from build123d import *

# Parameters (mm, degrees)
F0_W     = 35.4
F0_H     = 23.6
F1_DEPTH = 20
F3_DEPTH = 10


with BuildPart() as f1:
    # F0 (on Front) → F1 (new body)
    with BuildSketch(Plane.XZ):
        with Locations((-17.7, 28)):
            Rectangle(F0_W, F0_H)
        with BuildLine():
            ThreePointArc((0, -39.8), (39.8, 0), (0, 39.8))
            Line((0, 39.8), (0, 16.2))
            ThreePointArc((0, 16.2), (16.2, 0), (0, -16.2))
            Line((0, -16.2), (0, -39.8))
        make_face()
        with Locations((-17.7, -28)):
            Rectangle(F0_W, F0_H)
    extrude(amount=F1_DEPTH)

    # F2 (on face) → F3 (cut)
    with BuildSketch(Plane.XZ.offset(20)):
        with BuildLine():
            ThreePointArc((12.98208, 26.520214), (7.568156, 28.540833), (1.864359, 29.468293))
            ThreePointArc((1.864359, 29.468293), (-0.019794, 27.808362), (1.640137, 25.924209))
            ThreePointArc((1.640137, 25.924209), (6.657951, 25.108293), (11.420755, 23.330688))
            ThreePointArc((11.420755, 23.330688), (13.79618, 24.144789), (12.98208, 26.520214))
        make_face()
        with BuildLine():
            ThreePointArc((14.382505, 21.630955), (18.320101, 18.415444), (21.556008, 14.494592))
            ThreePointArc((21.556008, 14.494592), (24.020237, 14.01191), (24.502918, 16.476139))
            ThreePointArc((24.502918, 16.476139), (20.824632, 20.933009), (16.348729, 24.588111))
            ThreePointArc((16.348729, 24.588111), (13.887039, 24.092645), (14.382505, 21.630955))
        make_face()
        with BuildLine():
            ThreePointArc((23.271092, 11.541705), (25.073395, 6.788192), (25.915346, 1.77468))
            ThreePointArc((25.915346, 1.77468), (27.80809, 0.124552), (29.458219, 2.017296))
            ThreePointArc((29.458219, 2.017296), (28.501164, 7.716202), (26.45247, 13.119565))
            ThreePointArc((26.45247, 13.119565), (24.072851, 13.921324), (23.271092, 11.541705))
        make_face()
        with BuildLine():
            ThreePointArc((25.924209, -1.640137), (25.108293, -6.657951), (23.330688, -11.420755))
            ThreePointArc((23.330688, -11.420755), (24.144789, -13.79618), (26.520214, -12.98208))
            ThreePointArc((26.520214, -12.98208), (28.540833, -7.568156), (29.468293, -1.864359))
            ThreePointArc((29.468293, -1.864359), (27.808362, 0.019794), (25.924209, -1.640137))
        make_face()
        with BuildLine():
            ThreePointArc((21.630955, -14.382505), (18.415444, -18.320101), (14.494592, -21.556008))
            ThreePointArc((14.494592, -21.556008), (14.01191, -24.020237), (16.476139, -24.502918))
            ThreePointArc((16.476139, -24.502918), (20.933009, -20.824632), (24.588111, -16.348729))
            ThreePointArc((24.588111, -16.348729), (24.092645, -13.887039), (21.630955, -14.382505))
        make_face()
        with BuildLine():
            ThreePointArc((11.541705, -23.271092), (6.788192, -25.073395), (1.77468, -25.915346))
            ThreePointArc((1.77468, -25.915346), (0.124552, -27.80809), (2.017296, -29.458219))
            ThreePointArc((2.017296, -29.458219), (7.716202, -28.501164), (13.119565, -26.45247))
            ThreePointArc((13.119565, -26.45247), (13.921324, -24.072851), (11.541705, -23.271092))
        make_face()
    extrude(amount=-F3_DEPTH, mode=Mode.SUBTRACT)


solid = f1.part
Build history of the part. All positions in model axes, mm. A direction names the side the tool comes from. Give positions to 0.01 mm unless a question says otherwise; leave off trailing zeros. Order: outer loops, then holes, each group sorted by start corner. A loop starts at its lowest first (then second) coordinate and runs counter-clockwise, first axis right, second up. Notation, with made-up numbers: M 6.25,-22 L 39.25,-22 A16 ccw 39.25,6 Z; hole C 26,4.5 d8. An arc over 180 degrees is marked long. Use one line per item in the form item = value.
1) Drop flat-ended pins along their axis: pin 1 (8 mm diameter, centred on y = -15, z = 1, fed in from -X); pin 2 (10 mm diameter, centred on y = -3, z = 7.5, fed in from +X); pin 3 (5 mm diameter, centred on y = -17, z = 9, fed in from +X). Give the stop position or say it passes through.
Calculated:
pin_1 = 15.41
pin_2 = 39.72
pin_3 = 39.27
2) Two-plate mould, pull along Z, no slides. Class faces 1 (the face through (-35.4, -10, 28)), 2 (the face through (-18, -10, 39.8)), 3 (the face through (25.055, -15.07, 6.857)), 4 (the face through (27.16, -15.07, 0.2)): released by +Z, released by -Z, zero draft, split by the parting line, or undercut.
Calculated:
face_1 = zero draft
face_2 = released by +Z
face_3 = undercut
face_4 = undercut
3) Saw through at A-A (x = -15.5). Give the cut face in (y, z).
Calculated:
outline = M -20,-39.8 L 0,-39.8 L 0,-16.2 L -20,-16.2 Z; M -20,16.2 L 0,16.2 L 0,39.8 L -20,39.8 Z
4) Tool access for faces 5 (the face through (28.44, -15.07, -0.14)), 6 (the face through (16.196, -9.86, 0.356)): list every direction of +Z, -Z, +X, -X, +Y, -Y with a clear straight run to the whole face (end or side of a thin tool).
Calculated:
face_5 = -Y
face_6 = -X, +Y, -Y
5) Probe probe 1 along Z at (x, y) = (4, -13.5); probe 2 along Z at (x, y) = (-11, -8.5); probe 3 along Z at (x, y) = (2.5, -12.5). List the from-to ranges inside material, lowest first.
Calculated:
probe_1 = -39.6 to -29.26, -25.67 to -15.7, 15.7 to 25.67, 29.26 to 39.6
probe_2 = -39.8 to -16.2, 16.2 to 39.8
probe_3 = -39.72 to -29.42, -25.86 to -16.01, 16.01 to 25.86, 29.42 to 39.72
6) Saw through at C-C (y = -8.75). Give the cut face in (x, z), plus the area to 3 significant figures.
Calculated:
outline = M -35.4,-39.8 L 0,-39.8 A39.8 ccw 0,39.8 L -35.4,39.8 L -35.4,16.2 L 0,16.2 A16.2 cw 0,-16.2 L -35.4,-16.2 Z
area = 3,750 mm2
7) Saw through at B-B (y = -12.75). State how many separate pieces and enclosed holes the cut face has, plus the area to 3 significant figures.
Calculated:
separate_pieces = 1
enclosed_holes = 6
area = 3,460 mm2
